Could you check a few things on this model? Use its own coordinates, in mm. Face numbers are marked on the shaded views. A direction names the side the tool comes from. Round coordinates to 2 decimals unless told otherwise and drop trailing zeros. Loops run counter-clockwise (first coordinate to the right, second up) from the corner with the lowest first, then second, coordinate; pieces in that order, holes last. Notation, with made-up numbers: M 79.25,86.5 L 110.25,86.5 A11 cw 110.25,92.5 Z; hole C 71,74.25 d6. An arc over 180 degrees is marked long. One line per item, written item: value. Start each with the question number.
Q1. Imagine slicing it at A-A (z = 0). Give the number of separate pieces and of enclosed holes in the cut face, then the cut area to 3 significant figures.
Q2. I'm going to push flat-ended pins straight in: pin 1 Ø5 at (x, z) = (-0.5, 1) entering from +Y; pin 2 Ø3.5 at (x, z) = (-12.1, 0) entering from +Y; pin 3 Ø3 at (x, z) = (1, 0.5) entering from +Y; pin 4 Ø17.5 at (x, z) = (2, -0.5) entering from +Y. Where does each tip first touch, or does it pass through?
Q3. Thinking about a two-plate mould opening in X: for the marked faces 1, 2 and 3, which applies, released by +X, released by -X, zero draft, split by the parting line, or undercut?
Q4. Please list where these lines run through material, in increasing order: line 1 along X through (y, z) = (1.3, 0); line 2 along Y through (x, z) = (5, 0.5); line 3 along Z through (x, y) = (7.5, 3.6) (3 decimals).
Q5. Imagine slicing it at B-B (y = 1.8). Please give me the cut outline in (x, z).
Q6. Which directions (+Z, -Z, +X, -X, +Y, -Y) give clear straight access to the entire face, cutting with the end or side of a thin tool? Please do the marked faces 4 and 5.
from build123d import *

# Parameters (mm, degrees)
SKETCH1_R                                      = 15.15
BOSS_EXTRUDE1_DEPTH                            = 4
SKETCH4_R                                      = 8
CUT_EXTRUDE3_DEPTH                             = 1
SKETCH5_R                                      = 3
CUT_EXTRUDE4_DEPTH                             = 2.5
FILLET1_R                                      = 1
FILLET2_R                                      = 0.5
FILLET3_R                                      = 0.5
CUT_EXTRUDE5_START                             = -1.5
CUT_EXTRUDE5_DEPTH                             = 1.5
CSK_FOR_M2_5_FLAT_HEAD_MACHINE_SCREW1_AT_COUNT = 2
CSK_FOR_M2_5_FLAT_HEAD_MACHINE_SCREW1_AT_PITCH = 17.111984105
CSK_FOR_M2_5_FLAT_HEAD_MACHINE_SCREW_2_COUNT   = 2
CSK_FOR_M2_5_FLAT_HEAD_MACHINE_SCREW_2_PITCH   = 17.111984105
CSK_FOR_M2_5_FLAT_HEAD_MACHINE_SCREW_3_COUNT   = 2
CSK_FOR_M2_5_FLAT_HEAD_MACHINE_SCREW_3_PITCH   = 24.2


with BuildPart() as part:
    # Sketch1 → Boss-Extrude1 (new body)
    with BuildSketch(Plane(origin=(0, 0, 0), x_dir=(1, 0, 0), z_dir=(0, 1, 0))):
        with Locations(Location((0, 0, 0), (0, 0, 270))):
            Circle(SKETCH1_R)
    extrude(amount=BOSS_EXTRUDE1_DEPTH)

    # Sketch4 → Cut-Extrude3 (cut)
    with BuildSketch(Plane(origin=(0, 4, 0), x_dir=(1, 0, 0), z_dir=(0, 1, 0))):
        with Locations(Location((0, 0, 0), (0, 0, 270))):
            Circle(SKETCH4_R)
    extrude(amount=-CUT_EXTRUDE3_DEPTH, mode=Mode.SUBTRACT)

    # Sketch5 → Cut-Extrude4 (cut)
    with BuildSketch(Plane(origin=(0, 3, 0), x_dir=(1, 0, 0), z_dir=(0, 1, 0))):
        with Locations(Location((0, 0, 0), (0, 0, 270))):
            Circle(SKETCH5_R)
    extrude(amount=-CUT_EXTRUDE4_DEPTH, mode=Mode.SUBTRACT)

    # Fillet1
    fillet1_edges = [part.edges().sort_by_distance(p)[0] for p in [
        (0, 4, -8),
    ]]
    fillet(fillet1_edges, radius=FILLET1_R - 0.0001)  # a hair under: the kernel refuses the full size

    # Fillet2
    fillet2_edges = [part.edges().sort_by_distance(p)[0] for p in [
        (0, 3, -3),
    ]]
    fillet(fillet2_edges, radius=FILLET2_R)

    # Fillet3
    fillet3_edges = [part.edges().sort_by_distance(p)[0] for p in [
        (0, 4, -15.15),
    ]]
    fillet(fillet3_edges, radius=FILLET3_R)

    # Sketch2<2> → Cut-Extrude5 (cut)
    with BuildSketch(Plane(origin=(0, 4, 0), x_dir=(1, 0, 0), z_dir=(0, 1, 0)).offset(CUT_EXTRUDE5_START)):
        with BuildLine():
            Line((-12.1, 2.75), (-14.898322053, 2.75))
            ThreePointArc((-14.898322053, 2.75), (-15.15, 0), (-14.898322053, -2.75))
            Line((-14.898322053, -2.75), (-12.1, -2.75))
            ThreePointArc((-12.1, -2.75), (-9.35, 0), (-12.1, 2.75))
        make_face()
        with BuildLine():
            Line((-2.75, -12.1), (-2.75, -14.898322053))
            ThreePointArc((-2.75, -14.898322053), (0, -15.15), (2.75, -14.898322053))
            Line((2.75, -14.898322053), (2.75, -12.1))
            ThreePointArc((2.75, -12.1), (0, -9.35), (-2.75, -12.1))
        make_face()
        with BuildLine():
            ThreePointArc((15.15, 0), (15.086949312, 1.380746337), (14.898322053, 2.75))
            Line((14.898322053, 2.75), (12.1, 2.75))
            ThreePointArc((12.1, 2.75), (9.35, 0), (12.1, -2.75))
            Line((12.1, -2.75), (14.898322053, -2.75))
            ThreePointArc((14.898322053, -2.75), (15.086949312, -1.380746337), (15.15, 0))
        make_face()
        with BuildLine():
            ThreePointArc((-2.75, 12.1), (0, 9.35), (2.75, 12.1))
            Line((2.75, 12.1), (2.75, 14.898322053))
            ThreePointArc((2.75, 14.898322053), (0, 15.15), (-2.75, 14.898322053))
            Line((-2.75, 14.898322053), (-2.75, 12.1))
        make_face()
    extrude(amount=CUT_EXTRUDE5_DEPTH, mode=Mode.SUBTRACT)

    # Sketch7 → CSK for M2.5 Flat Head Machine Screw1 (revolve, cut)
    with BuildSketch(Plane(origin=(0, 2.5, -12.1), x_dir=(0, 0, 1), z_dir=(1, 0, 0))):
        Polygon((0, 0), (0, 2.5), (1.4, 2.5), (1.4, 1.35), (2.75, 0), align=None)
    csk_for_m2_5_flat_head_machine_screw1 = revolve(axis=Axis((0, 8.85, -12.1), (0, -1, 0)), mode=Mode.SUBTRACT)

    # CSK for M2.5 Flat Head Machine Screw1 at: CSK for M2.5 Flat Head Machine Screw1 ×2
    with Locations(*[Vector(-0.7071067811865512, 0, 0.7071067811865439) * (i * CSK_FOR_M2_5_FLAT_HEAD_MACHINE_SCREW1_AT_PITCH) for i in range(1, CSK_FOR_M2_5_FLAT_HEAD_MACHINE_SCREW1_AT_COUNT)]):
        add(csk_for_m2_5_flat_head_machine_screw1, mode=Mode.SUBTRACT)

    # CSK for M2.5 Flat Head Machine Screw 2: CSK for M2.5 Flat Head Machine Screw1 ×2
    with Locations(*[Vector(0.7071067811865464, 0, 0.7071067811865488) * (i * CSK_FOR_M2_5_FLAT_HEAD_MACHINE_SCREW_2_PITCH) for i in range(1, CSK_FOR_M2_5_FLAT_HEAD_MACHINE_SCREW_2_COUNT)]):
        add(csk_for_m2_5_flat_head_machine_screw1, mode=Mode.SUBTRACT)

    # CSK for M2.5 Flat Head Machine Screw 3: CSK for M2.5 Flat Head Machine Screw1 ×2
    with Locations(*[(0, 0, i * CSK_FOR_M2_5_FLAT_HEAD_MACHINE_SCREW_3_PITCH) for i in range(1, CSK_FOR_M2_5_FLAT_HEAD_MACHINE_SCREW_3_COUNT)]):
        add(csk_for_m2_5_flat_head_machine_screw1, mode=Mode.SUBTRACT)


solid = part.part
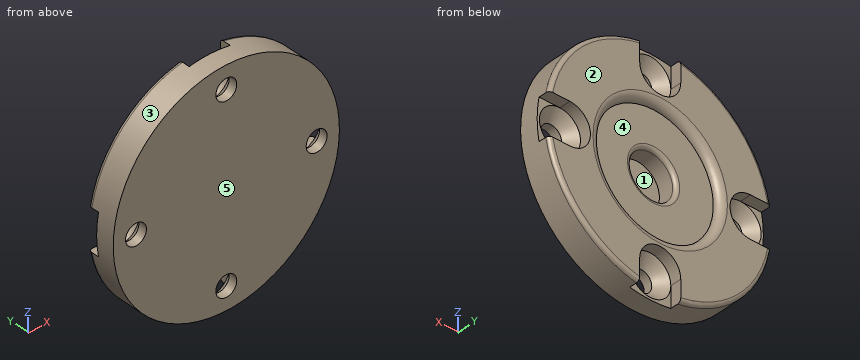
Report:
1. separate pieces: 3
1. enclosed holes: 0
1. area: 54.6 mm²
2. pin 1: stops at y = 3
2. pin 2: stops at y = 1.5
2. pin 3: stops at y = 0.5
2. pin 4: stops at y = 4
3. face 1: undercut
3. face 2: zero draft
3. face 3: split by the parting line
4. line 1: x = -15.15 to -13.65, -10.55 to -3, 3 to 10.55, 13.65 to 15.15
4. line 2: y = 0 to 3
4. line 3: z = -13.152 to -3.315, 3.315 to 13.152
5. outline: C 0,0 d30.3; hole C -12.1,0 d4.1; hole C 0,0 d6; hole C 0,-12.1 d4.1; hole C 0,12.1 d4.1; hole C 12.1,0 d4.1
6. face 4: +Y
6. face 5: +Z, -Z, +X, -X, -Y
